Solid Edge part; units mm, degrees
sketch "Sketch1" plane through (0, 0, 0) normal (0, 0, 1) x (1, 0, 0)
  line L0 (0, 0) -> (47.0718, 0)
  line L1 (47.0718, 0) -> (60, 7.4641)
  line L2 (60, 7.4641) -> (60, 25)
  line L3 (60, 25) -> (56, 25)
  line L4 (56, 25) -> (56, 9.7735)
  line L5 (56, 9.7735) -> (46, 4)
  line L6 (46, 4) -> (0, 4)
  line L7 (0, 0) -> (0, 4)
  dimension "D1" = 56
extrude "Protrusion1" add sketch "Sketch1" along normal blind 25
mirror "Mirror1" about plane through (0, 0, 0) normal (1, 0, 0) of "Protrusion1"
sketch "Sketch2" plane through (0, 0, 15) normal (0, -1, 0) x (1, 0, 0)
  line L0 (-43, -15) -> (-35, -23)
  line L1 (-35, -23) -> (35, -23)
  line L2 (35, -23) -> (43, -15)
  line L3 (43, -15) -> (-43, -15)
  dimension "D1" = 35
  dimension "D2" = 43
  dimension "D3" = 35
extrude "Protrusion2" add sketch "Sketch2" against normal up to vertex (4 mm away)
hole "Hole1" at (-30, 0, -4) direction (0, 1, 0) diameter 3.4 end up to next start chamfer 0.3 start chamfer angle 45 end chamfer 0.3 end chamfer angle 45
hole "Hole2" at (30, 0, -4) direction (0, 1, 0) diameter 3.4 end up to next start chamfer 0.3 start chamfer angle 45 end chamfer 0.3 end chamfer angle 45
sketch "Sketch3" plane through (0, 0, 8.5) normal (0, -1, 0) x (1, 0, 0)
  line L0 (-43, 16.5) -> (43, 16.5)
  line L1 (33.6676, 24.5) -> (43, 16.5)
  line L2 (-33.6676, 24.5) -> (33.6676, 24.5)
  line L3 (-43, 16.5) -> (-33.6676, 24.5)
extrude "Protrusion3" add sketch "Sketch3" against normal up to vertex (4 mm away)
hole "Hole3" at (-30, 0, 29) direction (0, 1, 0) diameter 3.4 end up to next start chamfer 0.3 start chamfer angle 45 end chamfer 0.3 end chamfer angle 45
hole "Hole4" at (30, 0, 29) direction (0, 1, 0) diameter 3.4 end up to next start chamfer 0.3 start chamfer angle 45 end chamfer 0.3 end chamfer angle 45
properties material "Polyethylene, low density"
The listing builds one solid part. Answer for the finished solid, in the listing's coordinates (mm). A direction names the side the tool comes from. Give positions to 0.01 mm unless a question says otherwise; leave off trailing zeros. Order: outer loops, then holes, each group sorted by start corner. A loop starts at its lowest first (then second) coordinate and runs counter-clockwise, first axis right, second up. Notation, with made-up numbers: (2.25, 56.5) - (47.25, 56.5) arc R25 ccw to (47.25, 70.5) - close; hole circle Ø7 at (33, 89). An arc over 180 degrees is marked (long way). Use one line per item in the form item = value.
1) Find section B-B on z = -4. Determine the outline of the cut face in (x, y), and give its area (3 significant figures).
Verdict:
outline = (-39, 0) - (-32, 0) - (-31.7, 0.3) - (-31.7, 3.7) - (-32, 4) - (-39, 4) - close; (-28.3, 0.3) - (-28, 0) - (28, 0) - (28.3, 0.3) - (28.3, 3.7) - (28, 4) - (-28, 4) - (-28.3, 3.7) - close; (31.7, 0.3) - (32, 0) - (39, 0) - (39, 4) - (32, 4) - (31.7, 3.7) - close
area = 284 mm^2
2) The mould has two halves that part along X. Classify faces 4 (the flat face through (-1, 0, 12)), 5 (the flat face through (-50.93, 6.846, 12.325)), 6 (the flat face through (-60, 16, 12)), 7 (the flat face through (-56, 17, 12)): released by +X, released by -X, zero draft, split by the parting line, or undercut.
Verdict:
face_4 = zero draft
face_5 = undercut
face_6 = released by -X
face_7 = undercut
3) For faces 1 (the flat face through (54, 8, 25)), 2 (the flat face through (53.445, 3.68, 12.325)), 3 (the flat face through (-55, 9, 0)), determine the directions among +Z, -Z, +X, -X, +Y, -Y from which every point of the face is accessible in a straight line to the end or side of a thin tool.
Verdict:
face_1 = +Z, +X, +Y, -Y
face_2 = +Z, -Z, +X, -Y
face_3 = -Z, -X, +Y, -Y
4) Consider probe 1 along Z at (x, y) = (30, 1.8); probe 2 along X at (y, z) = (23.75, 12); probe 3 along X at (y, z) = (2.2, 29). Determine where each line is inside the solid, lowest interval first. Write a range as [from, to].
Verdict:
probe_1 = [-8, -5.7], [-2.3, 27.3], [30.7, 33]
probe_2 = [-60, -56], [56, 60]
probe_3 = [-38.33, -31.7], [-28.3, 28.3], [31.7, 38.33]
5) Find section A-A on x = 30. Determine the outline of the cut face in (y, z).
Verdict:
outline = (0, -8) - (4, -8) - (4, -6) - (3.7, -5.7) - (0.3, -5.7) - (0, -6) - close; (0, -2) - (0.3, -2.3) - (3.7, -2.3) - (4, -2) - (4, 27) - (3.7, 27.3) - (0.3, 27.3) - (0, 27) - close; (0, 31) - (0.3, 30.7) - (3.7, 30.7) - (4, 31) - (4, 33) - (0, 33) - close
6) Find section C-C on y = 13. Determine the outline of the cut face in (x, z).
Verdict:
outline = (-60, 0) - (-56, 0) - (-56, 25) - (-60, 25) - close; (56, 0) - (60, 0) - (60, 25) - (56, 25) - close
7) Find section D-D on z = 14.5. Determine the outline of the cut face in (x, y), and give its area (3 significant figures).
Verdict:
outline = (-60, 7.46) - (-47.07, 0) - (47.07, 0) - (60, 7.46) - (60, 25) - (56, 25) - (56, 9.77) - (46, 4) - (-46, 4) - (-56, 9.77) - (-56, 25) - (-60, 25) - close
area = 609 mm^2
8) Each of these flat-tipped pins is pushed along its axis until it touches: pin 1 (1.5 mm diameter, centred on x = -44, z = 19, fed in from +Y); pin 2 (12 mm diameter, centred on x = 11.5, y = 15.5, fed in from +Z); pin 3 (13.5 mm diameter, centred on x = -55.5, y = 9, fed in from +Z); pin 4 (8.5 mm diameter, centred on x = -54, y = 15.5, fed in from -Z). Where does it stop, or does it pass through?
Verdict:
pin_1 = 4
pin_2 = through
pin_3 = 25
pin_4 = 0
